Check sheet for the modelled part. Datum: model origin and axes. Units: mm. Coordinates: 2 decimals unless noted, no trailing zeros. Write each loop counter-clockwise with the first axis right and the second up, starting at its lowest first coordinate (ties: lowest second). Pieces come first, ordered by that corner, then holes. Notation, with made-up numbers: M -36.5,61.25 L 15.5,61.25 A28 cw 15.5,80.25 Z; hole C -11,-1.5 d8. An arc over 180 degrees is marked long. Answer as CSV lines item,"result". Start each with the question number.
Q1. Sectioned sample at C-C, the plane x = 25. Record the cut outline in (y, z), then the cut area to 3 significant figures.
Q2. Depth check by flat-ended pin: pin 1 Ø1 at (y, z) = (-15.5, 117.5) entering from -X; pin 2 Ø3 at (x, z) = (24.5, 54.5) entering from +Y; pin 3 Ø2 at (x, y) = (7.5, 11.5) entering from +Z; pin 4 Ø6 at (x, y) = (-15, -15) entering from -Z. Enter the tip coordinate at first touch or a pass-through.
Q3. Sectioned sample at B-B, the plane y = -25. Record the cut outline in (x, z).
Q4. Thickness scan on line 1 along Y through (x, z) = (-25, 107); line 2 along Y through (x, z) = (15, 100); line 3 along Y through (x, z) = (25, 44). Record the ranges inside material, lowest first. Write a range as from..to.
Q5. Sectioned sample at A-A, the plane x = 3.5. Record the cut outline in (y, z), then the cut area to 3 significant figures.
Q6. Sectioned sample at D-D, the plane z = 29.5. Count the separate pieces of the cut face and the enclosed holes in it, then the cut area to 3 significant figures.
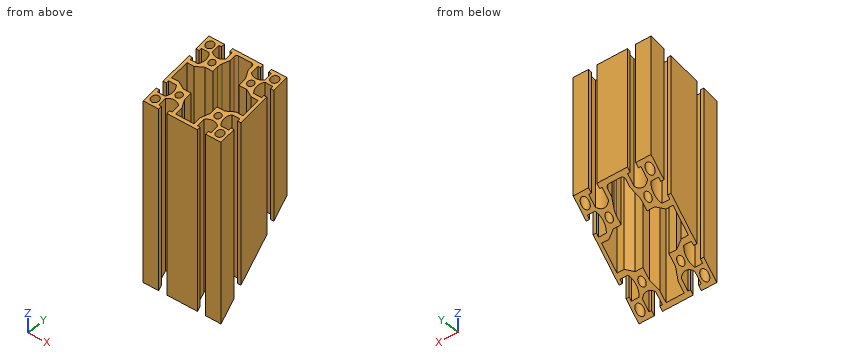
from build123d import *

# Parameters (mm, degrees)
F0_R          = 3
F0_R_2        = 2.5
F1_DEPTH      = 150
F2_R          = 2
F3_R          = 7
F6_DEPTH      = 30
F6_DEPTH_BACK = 30


# Not quite as in the source:
# - a feature names something its author has since deleted; it is built from what else it names


with BuildPart() as f1:
    # F0 (on Top) → F1 (new body)
    with BuildSketch(Plane.XY):
        with BuildLine():
            Line((18.15, -30), (30, -30))
            Line((30, -30), (30, -18.15))
            Line((30, -18.15), (27.5, -18.15))
            Line((27.5, -18.15), (27.5, -20.15))
            Line((27.5, -20.15), (21.5477069044, -20.15))
            ThreePointArc((21.5477069044, -20.15), (19.5, -15), (21.5477069044, -9.85))
            Line((21.5477069044, -9.85), (27.5, -9.85))
            Line((27.5, -9.85), (27.5, -11.85))
            Line((27.5, -11.85), (30, -11.85))
            Line((30, -11.85), (30, 11.85))
            Line((30, 11.85), (27.5, 11.85))
            Line((27.5, 11.85), (27.5, 9.85))
            Line((27.5, 9.85), (21.5477069044, 9.85))
            ThreePointArc((21.5477069044, 9.85), (19.5, 15), (21.5477069044, 20.15))
            Line((21.5477069044, 20.15), (27.5, 20.15))
            Line((27.5, 20.15), (27.5, 18.15))
            Line((27.5, 18.15), (30, 18.15))
            Line((30, 18.15), (30, 30))
            Line((30, 30), (18.15, 30))
            Line((18.15, 30), (18.15, 27.5))
            Line((18.15, 27.5), (20.15, 27.5))
            Line((20.15, 27.5), (20.15, 21.5477069044))
            ThreePointArc((20.15, 21.5477069044), (15, 19.5), (9.85, 21.5477069044))
            Line((9.85, 21.5477069044), (9.85, 27.5))
            Line((9.85, 27.5), (11.85, 27.5))
            Line((11.85, 27.5), (11.85, 30))
            Line((11.85, 30), (-11.85, 30))
            Line((-11.85, 30), (-11.85, 27.5))
            Line((-11.85, 27.5), (-9.85, 27.5))
            Line((-9.85, 27.5), (-9.85, 21.5477069044))
            ThreePointArc((-9.85, 21.5477069044), (-15, 19.5), (-20.15, 21.5477069044))
            Line((-20.15, 21.5477069044), (-20.15, 27.5))
            Line((-20.15, 27.5), (-18.15, 27.5))
            Line((-18.15, 27.5), (-18.15, 30))
            Line((-18.15, 30), (-30, 30))
            Line((-30, 30), (-30, 18.15))
            Line((-30, 18.15), (-27.5, 18.15))
            Line((-27.5, 18.15), (-27.5, 20.15))
            Line((-27.5, 20.15), (-21.5477069044, 20.15))
            ThreePointArc((-21.5477069044, 20.15), (-19.5, 15), (-21.5477069044, 9.85))
            Line((-21.5477069044, 9.85), (-27.5, 9.85))
            Line((-27.5, 9.85), (-27.5, 11.85))
            Line((-27.5, 11.85), (-30, 11.85))
            Line((-30, 11.85), (-30, -11.85))
            Line((-30, -11.85), (-27.5, -11.85))
            Line((-27.5, -11.85), (-27.5, -9.85))
            Line((-27.5, -9.85), (-21.5477069044, -9.85))
            ThreePointArc((-21.5477069044, -9.85), (-19.5, -15), (-21.5477069044, -20.15))
            Line((-21.5477069044, -20.15), (-27.5, -20.15))
            Line((-27.5, -20.15), (-27.5, -18.15))
            Line((-27.5, -18.15), (-30, -18.15))
            Line((-30, -18.15), (-30, -30))
            Line((-30, -30), (-18.15, -30))
            Line((-18.15, -30), (-18.15, -27.5))
            Line((-18.15, -27.5), (-20.15, -27.5))
            Line((-20.15, -27.5), (-20.15, -21.5477069044))
            ThreePointArc((-20.15, -21.5477069044), (-15, -19.5), (-9.85, -21.5477069044))
            Line((-9.85, -21.5477069044), (-9.85, -27.5))
            Line((-9.85, -27.5), (-11.85, -27.5))
            Line((-11.85, -27.5), (-11.85, -30))
            Line((-11.85, -30), (11.85, -30))
            Line((11.85, -30), (11.85, -27.5))
            Line((11.85, -27.5), (9.85, -27.5))
            Line((9.85, -27.5), (9.85, -21.5477069044))
            ThreePointArc((9.85, -21.5477069044), (15, -19.5), (20.15, -21.5477069044))
            Line((20.15, -21.5477069044), (20.15, -27.5))
            Line((20.15, -27.5), (18.15, -27.5))
            Line((18.15, -27.5), (18.15, -30))
        make_face()
        with Locations((-25, -25)):
            Circle(F0_R, mode=Mode.SUBTRACT)
        with Locations((-15, -15)):
            Circle(F0_R_2, mode=Mode.SUBTRACT)
        with Locations((25, -25)):
            Circle(F0_R, mode=Mode.SUBTRACT)
        with Locations((15, -15)):
            Circle(F0_R_2, mode=Mode.SUBTRACT)
        with Locations((-25, 25)):
            Circle(F0_R, mode=Mode.SUBTRACT)
        with Locations((-15, 15)):
            Circle(F0_R_2, mode=Mode.SUBTRACT)
        Polygon((-7, 22), (-7, 27.5), (0, 27.5), (7, 27.5), (7, 22), (10, 16), (10, 10), (16, 10), (22, 7), (27.5, 7), (27.5, 0), (27.5, -7), (22, -7), (16, -10), (10, -10), (10, -16), (7, -22), (7, -27.5), (0, -27.5), (-7, -27.5), (-7, -22), (-10, -16), (-10, -10), (-16, -10), (-22, -7), (-27.5, -7), (-27.5, 0), (-27.5, 7), (-22, 7), (-16, 10), (-10, 10), (-10, 16), align=None, mode=Mode.SUBTRACT)
        with Locations((15, 15)):
            Circle(F0_R_2, mode=Mode.SUBTRACT)
        with Locations((25, 25)):
            Circle(F0_R, mode=Mode.SUBTRACT)
    extrude(amount=F1_DEPTH)

    # F2
    f2_edges = [f1.edges().sort_by_distance(p)[0] for p in [
        (-7, 27.5, 75),
        (7, 27.5, 75),
    ]]
    fillet(f2_edges, radius=F2_R)

    # F3
    f3_edges = [f1.edges().sort_by_distance(p)[0] for p in [
        (-10, 16, 75),
        (10, 16, 75),
    ]]
    fillet(f3_edges, radius=F3_R)

    # F5 (on Right) → F6 (cut, two sides)
    with BuildSketch(Plane.YZ) as f6_sk:
        Polygon((115.2614038106, 44.5196963257), (64.8905500682, 94.8905500682), (-30, 0), (20.3708537424, -50.3708537424), align=None)
        Polygon((30, 150), (10.7683995954, 246.6837842107), (-148.7245392843, 214.9586661578), (-129.4929388797, 118.2748819471), align=None)
    extrude(amount=F6_DEPTH, mode=Mode.SUBTRACT)
    extrude(f6_sk.sketch, amount=-F6_DEPTH_BACK, mode=Mode.SUBTRACT)


solid = f1.part
Output:
1,outline,"M -30,0 L -28,2 L -28,138.46 L -30,138.07 Z; M -22,8 L -20.15,9.85 L -20.15,140.02 L -22,139.66 Z; M -9.85,20.15 L -7,23 L -7,142.64 L -9.85,142.07 Z; M 7,37 L 9.85,39.85 L 9.85,145.99 L 7,145.43 Z; M 20.15,50.15 L 22,52 L 22,148.41 L 20.15,148.04 Z; M 28,58 L 30,60 L 30,150 L 28,149.6 Z"
1,area,"1,530 mm^2"
2,pin 1,"stops at x = -19.57"
2,pin 2,"stops at y = 22.76"
2,pin 3,"passes through"
2,pin 4,"stops at z = 12"
3,outline,"M -30,5 L -28,5 L -28,139.06 L -30,139.06 Z; M -22,5 L -20.15,5 L -20.15,139.06 L -22,139.06 Z; M -9.85,5 L -7,5 L -7,139.06 L -9.85,139.06 Z; M 7,5 L 9.85,5 L 9.85,139.06 L 7,139.06 Z; M 20.15,5 L 22,5 L 22,139.06 L 20.15,139.06 Z; M 28,5 L 30,5 L 30,139.06 L 28,139.06 Z"
4,line 1,"y = -30..-28, -22..-20.15, -9.85..-7, 7..9.85, 20.15..22, 28..30"
4,line 2,"y = -19.5..-17.5, -12.5..-10, 10..12.5, 17.5..19.5"
4,line 3,"y = -30..-28, -22..-20.15, -9.85..-7, 7..9.85"
5,outline,"M -30,0 L -27.5,2.5 L -27.5,138.56 L -30,138.07 Z; M 27.5,57.5 L 30,60 L 30,150 L 27.5,149.5 Z"
5,area,"570 mm^2"
6,separate pieces,"1"
6,enclosed holes,"4"
6,area,"537 mm^2"
